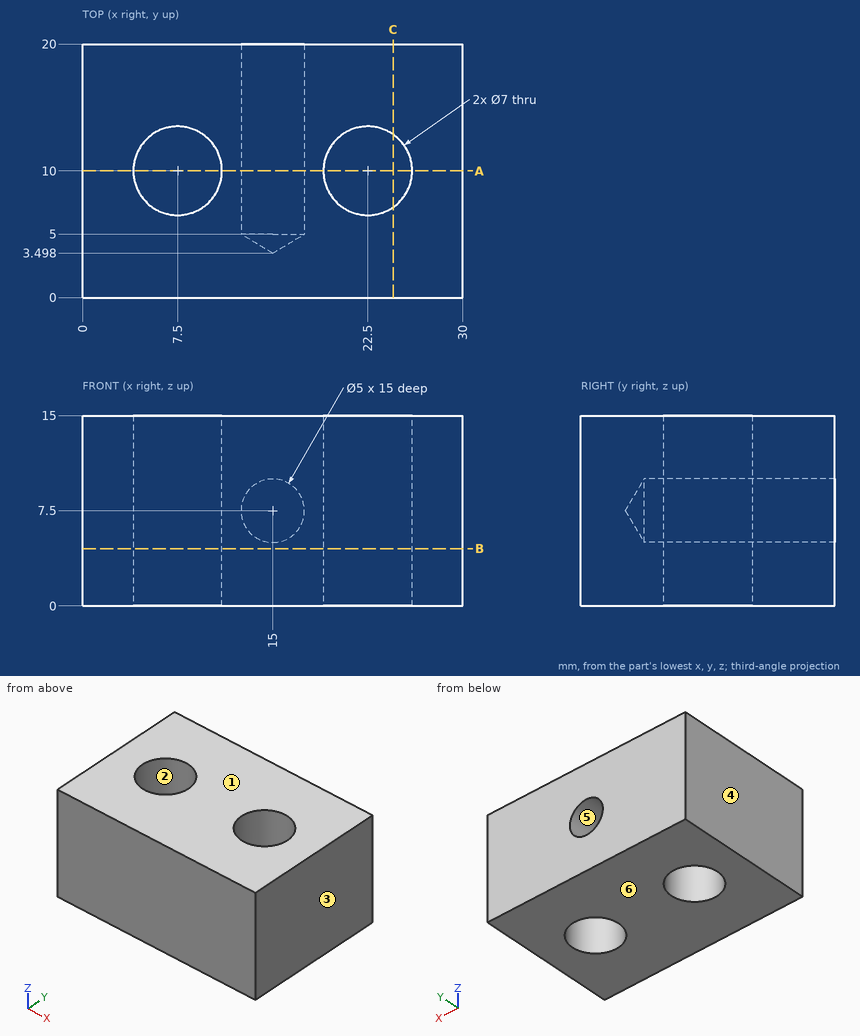
Geometry check sheet. Reference: drawing and pictorial views, mm from the part's lowest x, y, z. A direction names the side the tool comes from. Give positions to 0.01 mm unless a question says otherwise; leave off trailing zeros. Order: outer loops, then holes, each group sorted by start corner. A loop starts at its lowest first (then second) coordinate and runs counter-clockwise, first axis right, second up. Notation, with made-up numbers: M 75.5,57.5 L 98.5,57.5 A13 cw 98.5,72.5 Z; hole C -11,0.25 d9. An arc over 180 degrees is marked long. Answer in a Markdown table with one row per item. Add a question column.
Q1. Sectioned sample at B-B, the plane z = 4.5. Record the boundary of the cut face in (x, y), and give its area (3 significant figures).
Q2. Thickness scan on L1, parallel to Y at x = 7.5, z = 9; L2, parallel to X at y = 12.25, z = 7.25; L3, parallel to Z at x = 15, y = 12.75. Record the ranges inside material, lowest first.
Q3. Gauge pin test, flat end, axial feed: pin 1 Ø6.5 at (x, y) = (7.5, 10) entering from +Z. Record the tip position at first contact, or that the pin passes through.
Q4. Sectioned sample at C-C, the plane x = 24.5. Record the boundary of the cut face in (y, z), and give its area (3 significant figures).
Q5. Sectioned sample at A-A, the plane y = 10. Record the boundary of the cut face in (x, z), and give its area (3 significant figures).
Q6. Access from +Z, -Z, +X, -X, +Y, -Y to the whole of each face (thin tool, end or side, straight path). Record for the marked faces 5 and 6.
Q7. Release check for a two-part mould opening along X. For the marked faces 1, 2, 3 and 4 record: released by +X, released by -X, zero draft, split by the parting line, or undercut.
Verdict:
| question | item | result |
|---|---|---|
| 1 | outline | M 0,0 L 30,0 L 30,20 L 0,20 Z; hole C 7.5,10 d7; hole C 22.5,10 d7 |
| 1 | area | 523 mm² |
| 2 | L1 | 0 to 6.5, 13.5 to 20 |
| 2 | L2 | 0 to 4.82, 10.18 to 12.51, 17.49 to 19.82, 25.18 to 30 |
| 2 | L3 | 0 to 5, 10 to 15 |
| 3 | pin 1 | through |
| 4 | outline | M 0,0 L 7.13,0 L 7.13,15 L 0,15 Z; M 12.87,0 L 20,0 L 20,15 L 12.87,15 Z |
| 4 | area | 214 mm² |
| 5 | outline | M 0,0 L 4,0 L 4,15 L 0,15 Z; M 11,0 L 19,0 L 19,15 L 11,15 Z; M 26,0 L 30,0 L 30,15 L 26,15 Z; hole C 15,7.5 d5 |
| 5 | area | 220 mm² |
| 6 | face 5 | +Y |
| 6 | face 6 | -Z, +X, -X, +Y, -Y |
| 7 | face 1 | zero draft |
| 7 | face 2 | undercut |
| 7 | face 3 | released by +X |
| 7 | face 4 | released by -X |
